from build123d import *

# Parameters (mm, degrees)
SKETCH1_W           = 75
SKETCH1_H           = 3
BOSS_EXTRUDE1_DEPTH = 187.5
SKETCH2_R           = 4.9
BOSS_EXTRUDE2_DEPTH = 10
SKETCH3_W           = 7
SKETCH3_H           = 33
SKETCH3_W_2         = 2.5
SKETCH3_H_2         = 102.5
CUT_EXTRUDE1_DEPTH  = 1


with BuildPart() as part:
    # Sketch1 → Boss-Extrude1 (new body)
    with BuildSketch(Plane.XY):
        with Locations((37.5, 1.5)):
            Rectangle(SKETCH1_W, SKETCH1_H)
    extrude(amount=BOSS_EXTRUDE1_DEPTH)

    # Sketch2 → Boss-Extrude2 (add)
    with BuildSketch(Plane(origin=(0, 3, 0), x_dir=(1, 0, 0), z_dir=(0, 1, 0))):
        with Locations(Location((25, -177.5, 0), (0, 0, 90))):
            Circle(SKETCH2_R)
        with Locations(Location((45, -17.5, 0), (0, 0, 90))):
            Circle(SKETCH2_R)
    extrude(amount=BOSS_EXTRUDE2_DEPTH)

    # Sketch3 → Cut-Extrude1 (cut)
    with BuildSketch(Plane.XZ):
        with Locations((7.5, 26.5)):
            Rectangle(SKETCH3_W, SKETCH3_H)
        with Locations((7.5, 63.5)):
            Rectangle(SKETCH3_W, SKETCH3_H)
        with Locations((22.5, 26.5)):
            Rectangle(SKETCH3_W, SKETCH3_H)
        with Locations((22.5, 63.5)):
            Rectangle(SKETCH3_W, SKETCH3_H)
        with Locations((37.5, 26.5)):
            Rectangle(SKETCH3_W, SKETCH3_H)
        with Locations((37.5, 63.5)):
            Rectangle(SKETCH3_W, SKETCH3_H)
        with Locations((52.5, 26.5)):
            Rectangle(SKETCH3_W, SKETCH3_H)
        with Locations((52.5, 63.5)):
            Rectangle(SKETCH3_W, SKETCH3_H)
        with Locations((67.5, 26.5)):
            Rectangle(SKETCH3_W, SKETCH3_H)
        with Locations((67.5, 63.5)):
            Rectangle(SKETCH3_W, SKETCH3_H)
        with Locations((73.75, 136.25)):
            Rectangle(SKETCH3_W_2, SKETCH3_H_2)
    extrude(amount=-CUT_EXTRUDE1_DEPTH, mode=Mode.SUBTRACT)


solid = part.part
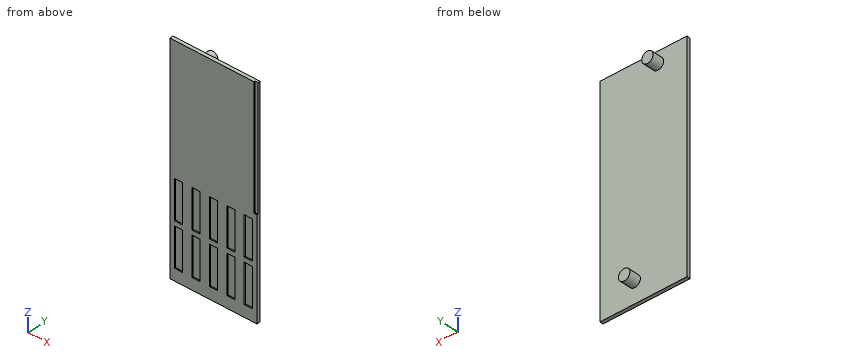
Model file for the job. Use its own axes, mm. Give positions to 0.01 mm unless a question says otherwise; leave off trailing zeros. Write each loop counter-clockwise with the first axis right and the second up, starting at its lowest first coordinate (ties: lowest second). Pieces come first, ordered by that corner, then holes. Notation, with made-up numbers: M 89.5,13 L 101.5,13 A11 cw 101.5,32 Z; hole C 63.25,46.25 d1. An arc over 180 degrees is marked long. One line per item, written item: value. Start each with the question number.
Q1. Saw through at B-B, the plane x = 6. Write the cut outline in (y, z).
Q2. Saw through at D-D, the plane x = 45. Write the cut outline in (y, z), plus the area to 4 significant figures.
Q3. Drop flat-ended pins along their axis: pin 1 Ø5 at (x, y) = (49, 8.5) entering from +Z; pin 2 Ø7.5 at (x, z) = (23, 65) entering from -Y; pin 3 Ø3 at (y, z) = (5.5, 122.5) entering from -X (3 decimals); pin 4 Ø3.5 at (x, z) = (6.5, 24.5) entering from -Y. Give the stop position or say it passes through.
Q4. Saw through at C-C, the plane y = 9. Write the cut outline in (x, z), plus the area to 3 significant figures.
Q5. Probe probe 1 along Z at (x, y) = (54, 0.5); probe 2 along Y at (x, z) = (52, 19); probe 3 along Y at (x, z) = (29, 113). List the from-to ranges inside material, lowest first. Write a range as [from, to].
Q6. Saw through at A-A, the plane z = 17.5. Write the cut outline in (x, y), plus the area to 3 significant figures.
Output values:
1. outline: M 0,0 L 3,0 L 3,187.5 L 0,187.5 L 0,80 L 1,80 L 1,47 L 0,47 L 0,43 L 1,43 L 1,10 L 0,10 Z
2. outline: M 0,0 L 3,0 L 3,12.6 L 13,12.6 L 13,22.4 L 3,22.4 L 3,187.5 L 0,187.5 Z
2. area: 660.5 mm²
3. pin 1: stops at z = 22.16
3. pin 2: stops at y = 0
3. pin 3: passes through
3. pin 4: stops at y = 1
4. outline: C 25,177.5 d9.8; C 45,17.5 d9.8
4. area: 151 mm²
5. probe 1: z = [0, 10], [43, 47], [80, 187.5]
5. probe 2: y = [1, 3]
5. probe 3: y = [0, 3]
6. outline: M 0,0 L 4,0 L 4,1 L 11,1 L 11,0 L 19,0 L 19,1 L 26,1 L 26,0 L 34,0 L 34,1 L 41,1 L 41,0 L 49,0 L 49,1 L 56,1 L 56,0 L 64,0 L 64,1 L 71,1 L 71,0 L 75,0 L 75,3 L 49.9,3 L 49.9,13 L 40.1,13 L 40.1,3 L 0,3 Z
6. area: 288 mm²
